Design review of the part built by this model. Coordinates are the model's own, in mm. A direction names the side the tool comes from. Give positions to 0.01 mm unless a question says otherwise; leave off trailing zeros. Write each loop counter-clockwise with the first axis right and the second up, starting at its lowest first coordinate (ties: lowest second). Pieces come first, ordered by that corner, then holes. Notation, with made-up numbers: (86.25, 26.25) -> (140.25, 26.25) arc R19 cw to (140.25, 55.25) -> close; hole circle Ø4 at (-21, 46.25). An arc over 180 degrees is marked (long way). Use CSV: the item, a comma, the result in double quotes.
```python
from build123d import *

# Parameters (mm, degrees)
F0_W     = 609.6
F0_H     = 152.4
F1_DEPTH = 25.4
F2_R     = 50.8
F3_DEPTH = 609.6
F4_W     = 609.6
F4_H     = 152.4
F4_R     = 50.8
F5_DEPTH = 25.4


with BuildPart() as f1:
    # F0 (on Top) → F1 (new body)
    with BuildSketch(Plane.XY):
        with Locations((-0.350654, 38.133061)):
            Rectangle(F0_W, F0_H)
    extrude(amount=F1_DEPTH)

    # F2 (on face) → F3 (join)
    with BuildSketch(Plane.XY.offset(25.4)):
        with Locations((215.54353, 35.826997)):
            Circle(F2_R)
        with Locations((63.145469, 36.595685)):
            Circle(F2_R)
        with Locations((-89.252593, 37.364373)):
            Circle(F2_R)
        with Locations((-241.650654, 38.133061)):
            Circle(F2_R)
    extrude(amount=F3_DEPTH)

    # F4 (on face) → F5 (join)
    with BuildSketch(Plane.XY.offset(635)):
        with Locations((-0.350654, 38.133061)):
            Rectangle(F4_W, F4_H)
        with Locations((-241.650654, 38.133061)):
            Circle(F4_R, mode=Mode.SUBTRACT)
    extrude(amount=-F5_DEPTH)


solid = f1.part
```
(1) Take a section at C-C (y = 49.5). Write out the cut boundary in (x, z), then the cut area to 3 significant figures.
Established:
outline,"(-305.15, 0) -> (304.45, 0) -> (304.45, 25.4) -> (264.47, 25.4) -> (264.47, 609.6) -> (304.45, 609.6) -> (304.45, 635) -> (-305.15, 635) -> (-305.15, 609.6) -> (-291.16, 609.6) -> (-291.16, 25.4) -> (-305.15, 25.4) -> close; hole (-192.14, 25.4) -> (-138.58, 25.4) -> (-138.58, 609.6) -> (-192.14, 609.6) -> close; hole (-39.92, 25.4) -> (14.01, 25.4) -> (14.01, 609.6) -> (-39.92, 609.6) -> close; hole (112.28, 25.4) -> (166.62, 25.4) -> (166.62, 609.6) -> (112.28, 609.6) -> close"
area,"261,000 mm2"
(2) Take a section at D-D (z = 71.5). Write out the cut boundary in (x, y), then the cut area to 3 significant figures.
Established:
outline,"circle Ø101.6 at (-241.65, 38.13); circle Ø101.6 at (-89.25, 37.36); circle Ø101.6 at (63.15, 36.6); circle Ø101.6 at (215.54, 35.83)"
area,"32,400 mm2"
(3) For line 1 along X through (y, z) = (39, 246); line 2 along Z through (x, y) = (2, 104); line 3 along X through (y, z) = (34.5, 312), list the stretches that pass through material, from the lowest coordinate up. Write a range as [from, to].
Established:
line 1,"x = [-292.44, -190.86], [-140.03, -38.48], [12.4, 113.89], [164.84, 266.24]"
line 2,"z = [0, 25.4], [609.6, 635]"
line 3,"x = [-292.32, -190.98], [-139.97, -38.53], [12.39, 113.9], [164.76, 266.33]"
(4) Take a section at B-B (x = 249). Write out the cut boundary in (y, z), then the cut area to 3 significant figures.
Established:
outline,"(-38.07, 0) -> (114.33, 0) -> (114.33, 25.4) -> (74.05, 25.4) -> (74.05, 609.6) -> (114.33, 609.6) -> (114.33, 635) -> (-38.07, 635) -> (-38.07, 609.6) -> (-2.4, 609.6) -> (-2.4, 25.4) -> (-38.07, 25.4) -> close"
area,"52,400 mm2"
(5) Tool access review of faces 1 (the face through (56.532, 86.963, 313.411)), 2 (the face through (-5, 114.333, 622)): name each direction out of +Z, -Z, +X, -X, +Y, -Y from which nothing blocks a thin tool from reaching the whole face with its end or side.
Established:
face 1,"none"
face 2,"+Z, -Z, +X, -X, +Y"
(6) Mouldability with a two-part tool opening along X and no side actions: class faces 3 (the face through (304.449, 37, 13)), 4 (the face through (-5, 39, 25.4)), 5 (the face through (-305.151, 37, 622)), 6 (the face through (-5, 114.333, 13)) as +X half, -X half, draft (parallel to the pull), parting line (faces both ways), or undercut.
Established:
face 3,"+X half"
face 4,"undercut"
face 5,"-X half"
face 6,"draft"
(7) Clearance check with flat-ended pins moving along their axes: pin 1 (2 mm diameter, centred on x = 69, z = 348.5, fed in from -Y); pin 2 (6 mm diameter, centred on y = -8, z = 399.5, fed in from +X); pin 3 (3 mm diameter, centred on y = 2.5, z = 289.5, fed in from -X). State where each tip first meets the part, or that it passes through.
Established:
pin 1,"stops at y = -13.97"
pin 2,"stops at x = 245.77"
pin 3,"stops at x = -279.27"
(8) Take a section at A-A (y = -25). Write out the cut boundary in (x, z), then the cut area to 3 significant figures.
Established:
outline,"(-305.15, 0) -> (304.45, 0) -> (304.45, 25.4) -> (-305.15, 25.4) -> close; (-305.15, 609.6) -> (304.45, 609.6) -> (304.45, 635) -> (-305.15, 635) -> close"
area,"31,000 mm2"
